from build123d import *

# Parameters (mm, degrees)
CBORE_FOR_M5_SHCS1_D           = 5.5
CBORE_FOR_M5_SHCS1_CBORE_D     = 9
CBORE_FOR_M5_SHCS1_CBORE_DEPTH = 2


with BuildPart() as part:
    # Sketch1 → Revolve1 (revolve)
    with BuildSketch(Plane(origin=(0, 0, 0), x_dir=(0, 0, -1), z_dir=(1, 0, 0)), mode=Mode.PRIVATE) as revolve1_sk:
        Polygon((0, -6.35), (0, 16), (-4, 16), (-4, 0), (-25, 0), (-25, -6.35), align=None)
    revolve(revolve1_sk.sketch.rotate(Axis((0, -6.35, 0), (0, 1, 0)), 180), axis=Axis((0, -6.35, 0), (0, 1, 0)))

    # CBORE for M5 SHCS1 (through all)
    with Locations(Plane(origin=(0, 0, 0), x_dir=(-1, 0, 0), z_dir=(0, 1, 0))):
        with Locations((0, -15.5), (13.423393759, 7.75), (-13.423393759, 7.75)):
            CounterBoreHole(CBORE_FOR_M5_SHCS1_D / 2, CBORE_FOR_M5_SHCS1_CBORE_D / 2, CBORE_FOR_M5_SHCS1_CBORE_DEPTH)


solid = part.part
Source: CAD feature listing. Evaluate the final solid. Frame: model axes, mm. A direction names the side the tool comes from. Coordinates: 2 decimals unless noted, no trailing zeros. Order: outer loops, then holes, each group sorted by start corner. A loop starts at its lowest first (then second) coordinate and runs counter-clockwise, first axis right, second up. Notation, with made-up numbers: M -39.5,-5.75 L -15.5,-5.75 A10 cw -15.5,9.25 Z; hole C 60.25,21.25 d8. An arc over 180 degrees is marked long. Write each question's results on one line, items separated by ' | '. Start each with the question number.
Item 1: Set-up query: faces 1 (the face through (-7.509, -3.219, -23.846)), 2 (the face through (0.59, -0.99, -11.04)). Return all of +Z, -Z, +X, -X, +Y, -Y with unobstructed straight access to the full face (end or side cutting, diameter ignored); none if empty.
Item 2: Draft query along Z for faces 3 (the face through (3.905, 7.888, 0.867)), 4 (the face through (0, 16, 0)), 5 (the face through (-11, -2, 6)). Return one class per face: pulls with the +Z half, pulls with the -Z half, needs draft (parallel to the pull), parting line crosses it, or undercut.
Item 3: Cut plane A-A (x = 0). Return loops of the section in (y, z), and give its area (3 significant figures).
Item 4: First-contact query: pin 1 Ø5 at (x, z) = (7, 0) entering from +Y; pin 2 Ø8 at (y, z) = (1.5, -11) entering from +X; pin 3 Ø4.5 at (x, z) = (-1, -15.5) entering from +Y. Flat tips, straight axial feed; report the tip coordinate or a pass-through.
Item 5: Line query: probe 1 along Y at (x, z) = (-0.5, -4); probe 2 along Z at (x, y) = (-1, -4.5); probe 3 along Z at (x, y) = (10, -1). Output: solid intervals per line, ascending.
Item 6: Cut plane B-B (z = 7.75). Return loops of the section in (x, y).
Item 7: Cut plane C-C (z = -15.5). Return loops of the section in (x, y), and give its area (3 significant figures).
Item 8: Cut plane D-D (z = 0). Return loops of the section in (x, y), and give its area (4 significant figures).
Checked values:
1) face 1: +Y, -Y | face 2: +Y
2) face 3: parting line crosses it | face 4: needs draft | face 5: undercut
3) outline: M -6.35,-25 L 0,-25 L 0,-20 L -2,-20 L -2,-18.25 L -6.35,-18.25 Z; M -6.35,-12.75 L -2,-12.75 L -2,-11 L 0,-11 L 0,-4 L 16,-4 L 16,4 L 0,4 L 0,25 L -6.35,25 Z | area: 404 mm2
4) pin 1: stops at y = 0 | pin 2: stops at x = 23.91 | pin 3: stops at y = -2
5) probe 1: y = -6.35 to 0 | probe 2: z = -24.98 to -18.06, -12.94 to 24.98 | probe 3: z = -22.91 to 4.83, 10.67 to 22.91
6) outline: M -23.77,-6.35 L -16.17,-6.35 L -16.17,-2 L -17.92,-2 L -17.92,0 L -23.77,0 Z; M -10.67,-6.35 L 10.67,-6.35 L 10.67,-2 L 8.92,-2 L 8.92,0 L -8.92,0 L -8.92,-2 L -10.67,-2 Z; M 16.17,-6.35 L 23.77,-6.35 L 23.77,0 L 17.92,0 L 17.92,-2 L 16.17,-2 Z
7) outline: M -19.62,-6.35 L -2.75,-6.35 L -2.75,-2 L -4.5,-2 L -4.5,0 L -19.62,0 Z; M 2.75,-6.35 L 19.62,-6.35 L 19.62,0 L 4.5,0 L 4.5,-2 L 2.75,-2 Z | area: 207 mm2
8) outline: M -25,-6.35 L 25,-6.35 L 25,0 L 4,0 L 4,16 L -4,16 L -4,0 L -25,0 Z | area: 445.5 mm2
